The figure shows three views and two pictorial views of one solid part (mm, origin at its lowest corner). Answer the questions. A direction names the side the tool comes from. Round coordinates to 2 decimals unless told otherwise and drop trailing zeros. Write each loop counter-clockwise with the first axis right and the second up, starting at its lowest first coordinate (ties: lowest second). Pieces come first, ordered by that corner, then holes.
Item 1: A tool of negligible diameter and unlimited length cuts with its end or side. For the marked faces 5, 6, 7 and 8, from which of +Z, -Z, +X, -X, +Y, -Y can it reach the whole face along a straight path? Write none if from no direction.
Item 2: For a pull along X with two mould halves and no side action, classify the marked faces 1, 2, 3 and 4 as +X half, -X half, draft (parallel to the pull), parting line (faces both ways), or undercut.
Item 3: Each of these flat-tipped pins is pushed along its axis until it touches: pin 1 (15 mm diameter, centred on x = 64, y = 20, fed in from -Z); pin 2 (11 mm diameter, centred on x = 82, z = 13, fed in from +Y); pin 3 (18 mm diameter, centred on x = 50, y = 25, fed in from -Z); pin 4 (9.5 mm diameter, centred on x = 50, y = 25, fed in from +Z). Where does it stop, or does it pass through?
Item 4: Find section D-D on y = 32. Give the vertices of the cut face in (x, z), then the cut area to 3 significant figures.
Item 5: Find section B-B on z = 5.5. Give the vertices of the cut face in (x, y).
Item 6: Find section A-A on y = 25. Give the vertices of the cut face in (x, z), then the cut area to 3 significant figures.
Item 7: Find the intervals of material crossed by probe 1 along Y at (x, z) = (50, 19.35); probe 2 along Y at (x, z) = (50, 17); probe 3 along X at (y, z) = (25, 18.7), in increasing order.
Item 8: Find section C-C on x = 40. Give the vertices of the cut face in (y, z).
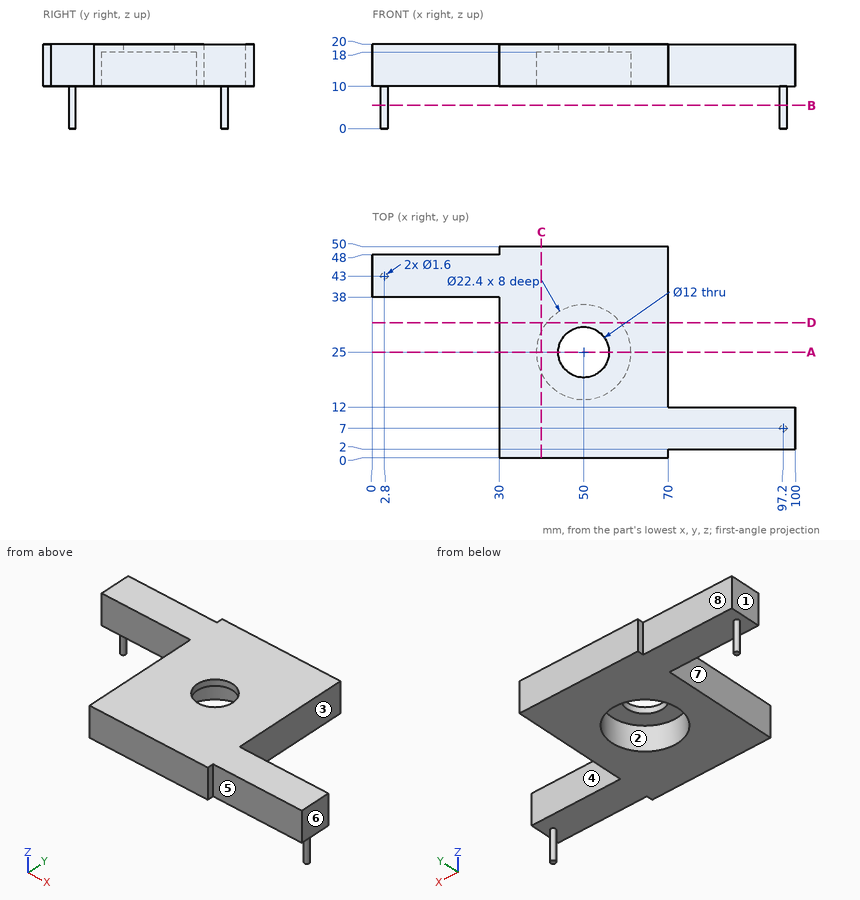
Check values:
1. face 5: +Z, -Z, +X, -Y
1. face 6: +Z, -Z, +X, +Y, -Y
1. face 7: +Z, -Z, -X, -Y
1. face 8: +Z, -Z, -X, +Y
2. face 1: -X half
2. face 2: undercut
2. face 3: +X half
2. face 4: draft
3. pin 1: stops at z = 10
3. pin 2: stops at y = 12
3. pin 3: stops at z = 18
3. pin 4: passes through
4. outline: (30, 10) - (41.26, 10) - (41.26, 18) - (58.74, 18) - (58.74, 10) - (70, 10) - (70, 20) - (30, 20) - close
4. area: 260 mm2
5. outline: circle Ø1.6 at (2.8, 43); circle Ø1.6 at (97.2, 7)
6. outline: (30, 10) - (38.8, 10) - (38.8, 18) - (44, 18) - (44, 20) - (30, 20) - close; (56, 18) - (61.2, 18) - (61.2, 10) - (70, 10) - (70, 20) - (56, 20) - close
6. area: 197 mm2
7. probe 1: y = 0 to 19, 31 to 50
7. probe 2: y = 0 to 13.8, 36.2 to 50
7. probe 3: x = 30 to 44, 56 to 70
8. outline: (0, 10) - (19.96, 10) - (19.96, 18) - (30.04, 18) - (30.04, 10) - (50, 10) - (50, 20) - (0, 20) - close
